from build123d import *

# Parameters (mm, degrees)
SKETCH_W        = 50
SKETCH_H        = 56
PAD_DEPTH       = 12
SKETCH001_R     = 16.2
POCKET_DEPTH    = 12.001
POCKET001_DEPTH = 56.001
SKETCH003_W     = 3
SKETCH003_H     = 6
POCKET002_DEPTH = 50.001
SKETCH004_W     = 72.31723
SKETCH004_H     = 2
POCKET003_DEPTH = 11.9
SKETCH005_W     = 25.040878
SKETCH005_H     = 17.68627
SKETCH005_W_2   = 12.208063
SKETCH005_H_2   = 50.590956
POCKET004_DEPTH = 5


with BuildPart() as part:
    # Sketch → Pad (new body)
    with BuildSketch(Plane.XY):
        Rectangle(SKETCH_W, SKETCH_H)
    extrude(amount=PAD_DEPTH)

    # Sketch001 → Pocket (cut, through all)
    with BuildSketch(Plane.XY.offset(12)):
        with Locations((0, -7.8)):
            Circle(SKETCH001_R)
    extrude(amount=-POCKET_DEPTH, mode=Mode.SUBTRACT)

    # Sketch002 → Pocket001 (cut, through all)
    with BuildSketch(Plane.XZ.offset(28)):
        Polygon((-22.5, 6), (-20.237258, 8.262742), (-17.974517, 6), (-20.237258, 3.737258), align=None)
        Polygon((17.974517, 6), (20.237258, 8.262742), (22.5, 6), (20.237258, 3.737258), align=None)
    extrude(amount=-POCKET001_DEPTH, mode=Mode.SUBTRACT)

    # Sketch003 → Pocket002 (cut, through all)
    with BuildSketch(Plane.YZ.offset(25)):
        with Locations((-0.5, 6)):
            Rectangle(SKETCH003_W, SKETCH003_H)
    extrude(amount=-POCKET002_DEPTH, mode=Mode.SUBTRACT)

    # Sketch004 → Pocket003 (cut)
    with BuildSketch(Plane.XY.offset(12)):
        with Locations((1.135831, -7.756839)):
            Rectangle(SKETCH004_W, SKETCH004_H)
    extrude(amount=-POCKET003_DEPTH, mode=Mode.SUBTRACT)

    # Sketch005 → Pocket004 (cut)
    with BuildSketch(Plane.XZ.offset(28)):
        with Locations((-27.520439, 4.662494)):
            Rectangle(SKETCH005_W, SKETCH005_H)
        with Locations((21.104031, -3.872155)):
            Rectangle(SKETCH005_W_2, SKETCH005_H_2)
    extrude(amount=-POCKET004_DEPTH, mode=Mode.SUBTRACT)


solid = part.part
Can you work these out from the model? Positions are in its coordinate system, mm. A direction names the side the tool comes from. Give positions to 0.01 mm unless a question says otherwise; leave off trailing zeros. Write each loop counter-clockwise with the first axis right and the second up, starting at its lowest first coordinate (ties: lowest second). Pieces come first, ordered by that corner, then holes. Notation, with made-up numbers: (68.5, 86.5) -> (92.5, 86.5) arc R30 cw to (92.5, 116.5) -> close; hole circle Ø6 at (74.25, -22). An arc over 180 degrees is marked (long way). Answer as a JSON object with one key per item and string values. Group by question number.
Item 1: For faces 4 (the face through (19, -1, 9)), 5 (the face through (15, -26, 6)), 6 (the face through (-22, -6.757, 7)), 7 (the face through (21.4, -4.4, 4.9)), which set-ups out of +Z, -Z, +X, -X, +Y, -Y let a thin tool reach every point of the face, with its end or its side?
Item 2: Suppose I cut it at D-D (y = -16.5). Please give me the cut outline in (x, z).
Item 3: Suppose I cut it at B-B (y = -7.8). Please give me the cut outline in (x, z).
Item 4: We'd pull the mould along Z, two halves only. Please class faces 1 (the face through (-15, -26, 6)), 2 (the face through (-19.122, 14.311, 7.147)), 3 (the face through (21.4, -4.4, 7.1)): +Z half, -Z half, draft (parallel to the pull), parting line (faces both ways), or undercut.
Item 5: Suppose I cut it at A-A (z = 2.25). Please give me the cut outline in (x, y), plus the area to 3 significant figures.
Item 6: Suppose I cut it at C-C (x = -3.5). Please give me the cut outline in (y, z).
Item 7: I'm going to push flat-ended pins straight in: P1, Ø7, axis at x = -21.5, z = 6.5, coming from the -Y side; P2, Ø1.5, axis at y = -26, z = 8.5, coming from the -X side. Where does each tip first touch, or does it pass through?
Item 8: Please list where these lines run through material, in increasing order: line 1 (Y direction, x = 0, z = 8.25); line 2 (Y direction, x = 21, z = 9.75); line 3 (Z direction, x = -22, y = -5.5). Write a range as [from, to].
Findings:
{
 "1": {"face 4": "+X, -X", "face 5": "+Z, -Z, +X, -Y", "face 6": "+Z, +X, -X", "face 7": "+Y, -Y"},
 "2": {"outline": "(-25, 0) -> (-13.67, 0) -> (-13.67, 12) -> (-25, 12) -> close; (13.67, 0) -> (25, 0) -> (25, 12) -> (13.67, 12) -> close; hole (-22.5, 6) -> (-20.24, 3.74) -> (-17.97, 6) -> (-20.24, 8.26) -> close; hole (17.97, 6) -> (20.24, 3.74) -> (22.5, 6) -> (20.24, 8.26) -> close"},
 "3": {"outline": "(-25, 0) -> (-16.2, 0) -> (-16.2, 0.1) -> (-25, 0.1) -> close; (16.2, 0) -> (25, 0) -> (25, 0.1) -> (16.2, 0.1) -> close"},
 "4": {"face 1": "draft", "face 2": "undercut", "face 3": "undercut"},
 "5": {"outline": "(-25, -23) -> (-15, -23) -> (-15, -28) -> (15, -28) -> (15, -23) -> (25, -23) -> (25, -8.76) -> (16.17, -8.76) arc R16.2 cw to (-16.17, -8.76) -> (-25, -8.76) -> close; (-25, -6.76) -> (-16.17, -6.76) arc R16.2 cw to (16.17, -6.76) -> (25, -6.76) -> (25, 28) -> (-25, 28) -> close", "area": "1,840 mm²"},
 "6": {"outline": "(-28, 0) -> (-23.62, 0) -> (-23.62, 12) -> (-28, 12) -> close; (8.02, 0) -> (28, 0) -> (28, 12) -> (8.02, 12) -> close"},
 "7": {"P1": "stops at y = -23", "P2": "stops at x = -15"},
 "8": {"line 1": "y = [-28, -24], [8.4, 28]", "line 2": "y = [-23, -8.76], [-6.76, 28]", "line 3": "z = [0, 5.5], [6.5, 12]"}
}
